```python
from build123d import *

# Parameters (mm, degrees)
SKETCH2_R               = 2.5
CUT_EXTRUDE1_DEPTH      = 17
CUT_EXTRUDE1_DEPTH_BACK = 17
SKETCH3_R               = 10
CUT_EXTRUDE2_DEPTH      = 24
SKETCH4_R               = 13
CUT_EXTRUDE3_DEPTH      = 10


with BuildPart() as part:
    # Sketch1 → Revolve1 (revolve)
    with BuildSketch(Plane.XY):
        with BuildLine():
            Line((0, 16), (0, -16))
            Line((0, -16), (16, -16))
            Line((16, -16), (16, 5))
            Line((16, 5), (14.5, 5))
            Line((14.5, 5), (14.5, 6.5))
            Line((14.5, 6.5), (16, 6.5))
            Line((16, 6.5), (16, 9.5))
            Line((16, 9.5), (14.5, 9.5))
            Line((14.5, 9.5), (14.5, 11))
            Line((14.5, 11), (16, 11))
            Line((16, 11), (16, 13.487300546))
            Line((16, 13.487300546), (3.472963553, 15.69615506))
            ThreePointArc((3.472963553, 15.69615506), (1.743114855, 15.923893962), (0, 16))
        make_face()
    revolve(axis=Axis((0, 16, 0), (0, -1, 0)))

    # Sketch2 → Cut-Extrude1 (cut, two sides)
    with BuildSketch(Plane.XY) as cut_extrude1_sk:
        Circle(SKETCH2_R)
    extrude(amount=CUT_EXTRUDE1_DEPTH, mode=Mode.SUBTRACT)
    extrude(cut_extrude1_sk.sketch, amount=-CUT_EXTRUDE1_DEPTH_BACK, mode=Mode.SUBTRACT)

    # Sketch3 → Cut-Extrude2 (cut)
    with BuildSketch(Plane.XZ.offset(16)):
        Circle(SKETCH3_R)
    extrude(amount=-CUT_EXTRUDE2_DEPTH, mode=Mode.SUBTRACT)

    # Sketch4 → Cut-Extrude3 (cut)
    with BuildSketch(Plane.XZ.offset(16)):
        Circle(SKETCH4_R)
    extrude(amount=-CUT_EXTRUDE3_DEPTH, mode=Mode.SUBTRACT)


solid = part.part
```
The model under review builds one solid part; all positions refer to its coordinate system, in mm. A direction names the side the tool comes from. Round coordinates to 2 decimals unless told otherwise and drop trailing zeros. Write each loop counter-clockwise with the first axis right and the second up, starting at its lowest first coordinate (ties: lowest second). Pieces come first, ordered by that corner, then holes. Notation, with made-up numbers: (35.25, 86.25) - (67.25, 86.25) arc R20 ccw to (67.25, 110.25) - close; hole circle Ø3 at (-33.75, -4). An arc over 180 degrees is marked (long way). Answer as CSV lines item,"result". Start each with the question number.
(1) Draft analysis for pull direction Z (two halves, no side actions). For faces 4 (the flat face through (3.6, 6.5, 14.3)), 5 (the cylindrical face through (-3.47, -5.35, -15.62)), 6 (the flat face through (0, 8, 0)), 7 (the cylindrical face through (-10.316, -11.07, -7.91)), state which applies: pulls with the +Z half, pulls with the -Z half, needs draft (parallel to the pull), parting line crosses it, or undercut.
(2) For faces 1 (the cylindrical face through (9.237, 0.902, -3.83)), 2 (the cylindrical face through (2.385, 0.751, 12.795)), 3 (the flat face through (3.6, 11, 14.3)), list the 3-axis set-ups (+Z, -Z, +X, -X, +Y, -Y) from which the entire face can be reached by the end or side of a thin tool; tool diameter is ignored.
(3) For pin 1 Ø10 at (x, y) = (-8.5, -0.5) entering from -Z; pin 2 Ø6 at (x, y) = (-8.5, 6) entering from -Z; pin 3 Ø1.5 at (y, z) = (-0.5, -6) entering from +X, all flat-tipped, find the tip position at first contact; note any pin that passes through.
(4) We need section B-B on y = 1. State the section outline as (x, z) points, plus the area to 3 significant figures.
(5) We need section C-C on x = 0. Give the number of separate pieces and of enclosed holes in the cut face, plus the area to 3 significant figures.
(6) We need section D-D on y = -5. State the section outline as (x, z) points.
(7) To check wall thickness, follow line 1 (Z direction, x = 0, y = 4.25); line 2 (Z direction, x = 0, y = -11.25); line 3 (X direction, y = -3.5, z = -0.5). State the ranges of each line that lie inside material, in increasing order.
Worked answers:
1,face 4,"needs draft"
1,face 5,"parting line crosses it"
1,face 6,"undercut"
1,face 7,"undercut"
2,face 1,"-Y"
2,face 2,"+Z, -Z"
2,face 3,"none"
3,pin 1,"z = -15.61"
3,pin 2,"z = -15.01"
3,pin 3,"x = 15.11"
4,outline,"(-2.29, -15.84) - (-2.29, -9.73) arc R10 cw to (-2.29, 9.73) - (-2.29, 15.84) arc R16 ccw to start; (2.29, -15.84) arc R16 ccw to (2.29, 15.84) - (2.29, 9.73) arc R10 cw to (2.29, -9.73) - close"
4,area,"435 mm²"
5,separate pieces,"3"
5,enclosed holes,"0"
5,area,"379 mm²"
6,outline,"circle Ø32 at (0, 0); hole circle Ø20 at (0, 0)"
7,line 1,"-16 to -10, 10 to 16"
7,line 2,"-16 to -13, 13 to 16"
7,line 3,"-15.99 to -9.99, 9.99 to 15.99"
